Could you check a few things on this drawing? It's one solid part, dimensions in mm from its lowest x, y, z. A direction names the side the tool comes from. Round coordinates to 2 decimals unless told otherwise and drop trailing zeros. Write each loop counter-clockwise with the first axis right and the second up, starting at its lowest first coordinate (ties: lowest second). Pieces come first, ordered by that corner, then holes. Notation, with made-up numbers: (13.5, 61) -> (37.5, 61) arc R11 cw to (37.5, 72) -> close; hole circle Ø1 at (-35, 8.25). An arc over 180 degrees is marked (long way). Answer in a Markdown table with one row per item.
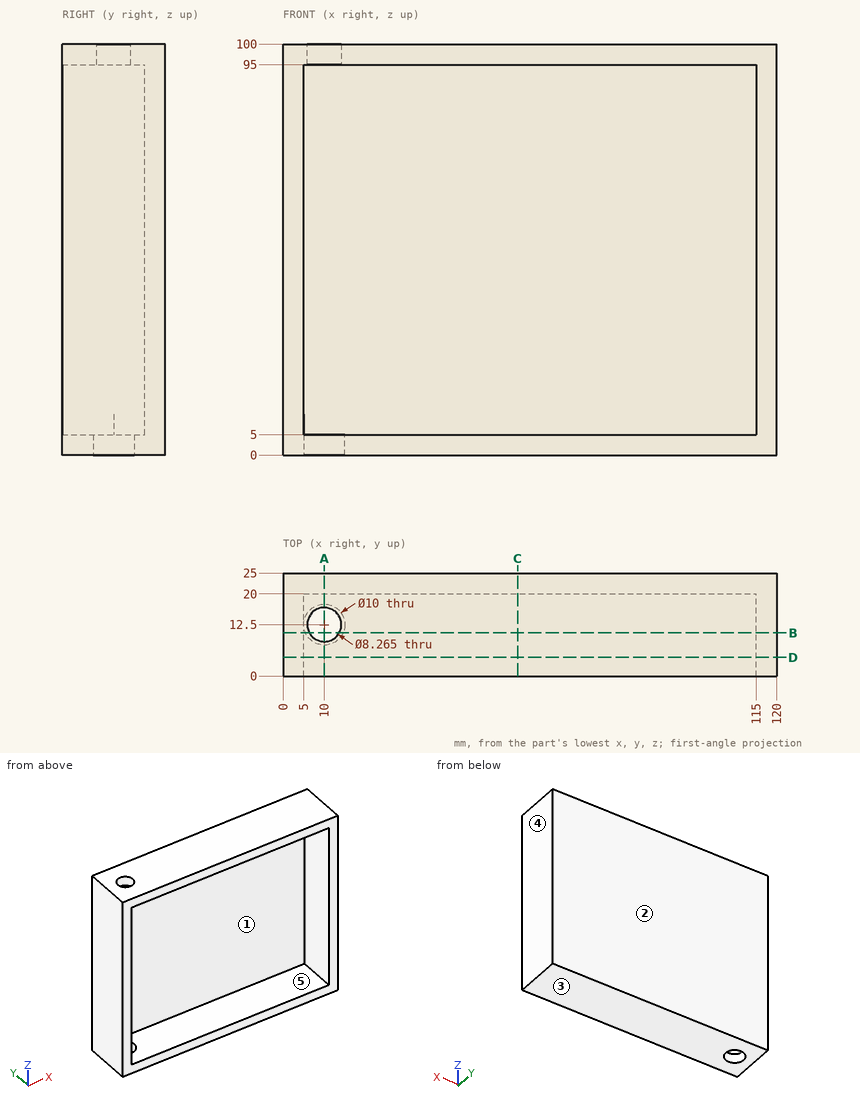
1) I want a section at B-B, the plane y = 10.5. List the corners of the cut face in (x, z) for me.
Response:
| item | result |
|---|---|
| outline | (0, 0) -> (5.42, 0) -> (5.42, 5) -> (5, 5) -> (5, 95) -> (6.38, 95) -> (6.38, 100) -> (0, 100) -> close; (13.62, 95) -> (115, 95) -> (115, 5) -> (14.58, 5) -> (14.58, 0) -> (120, 0) -> (120, 100) -> (13.62, 100) -> close |
2) I want a section at A-A, the plane x = 10. List the corners of the cut face in (y, z) for me.
Response:
| item | result |
|---|---|
| outline | (0, 0) -> (7.5, 0) -> (7.5, 5) -> (0, 5) -> close; (0, 95) -> (8.37, 95) -> (8.37, 100) -> (0, 100) -> close; (16.63, 95) -> (20, 95) -> (20, 5) -> (17.5, 5) -> (17.5, 0) -> (25, 0) -> (25, 100) -> (16.63, 100) -> close |
3) Which directions (+Z, -Z, +X, -X, +Y, -Y) give clear straight access to the entire face, cutting with the end or side of a thin tool? Please do the marked faces 1 and 2.
Response:
| item | result |
|---|---|
| face 1 | -Y |
| face 2 | +Z, -Z, +X, -X, +Y |
4) I want a section at D-D, the plane y = 4.5. List the corners of the cut face in (x, z) for me.
Response:
| item | result |
|---|---|
| outline | (0, 0) -> (120, 0) -> (120, 100) -> (0, 100) -> close; hole (5, 5) -> (115, 5) -> (115, 95) -> (5, 95) -> close |
5) I need wall thicknesses on line 1 (Y direction, x = 10, z = 97.8); line 2 (X direction, y = 12.5, z = 2.6); line 3 (X direction, y = 19.25, z = 85). Which ranges of each line are inside material? Lowest first, please. Write a range as [from, to].
Response:
| item | result |
|---|---|
| line 1 | y = [0, 8.37], [16.63, 25] |
| line 2 | x = [0, 5], [15, 120] |
| line 3 | x = [0, 5], [115, 120] |
6) We'd pull the mould along X, two halves only. Please class the marked faces 3, 4 and 5: +X half, -X half, draft (parallel to the pull), parting line (faces both ways), or undercut.
Response:
| item | result |
|---|---|
| face 3 | draft |
| face 4 | +X half |
| face 5 | undercut |
7) For pin 1 (1.5 mm diameter, centred on x = 86.5, z = 77.5, fed in from -Y), with a flat end and sliding along its axis, tell me the tip position at first contact or that it passes through.
Response:
| item | result |
|---|---|
| pin 1 | stops at y = 20 |
8) I want a section at C-C, the plane x = 57. List the corners of the cut face in (y, z) for me.
Response:
| item | result |
|---|---|
| outline | (0, 0) -> (25, 0) -> (25, 100) -> (0, 100) -> (0, 95) -> (20, 95) -> (20, 5) -> (0, 5) -> close |
